```python
from build123d import *

# Parameters (mm, degrees)
SKETCH1_R           = 292.1
BOSS_EXTRUDE1_DEPTH = 127
FILLET1_R           = 38.1
SKETCH2_R           = 15.875
CUT_EXTRUDE1_DEPTH  = 128


with BuildPart() as part:
    # Sketch1 → Boss-Extrude1 (new body)
    with BuildSketch(Plane(origin=(0, 0, 0), x_dir=(1, 0, 0), z_dir=(0, 1, 0))):
        Circle(SKETCH1_R)
    extrude(amount=BOSS_EXTRUDE1_DEPTH)

    # Fillet1
    fillet1_edges = [part.edges().sort_by_distance(p)[0] for p in [
        (-292.1, 0, 0),
        (-292.1, 127, 0),
    ]]
    fillet(fillet1_edges, radius=FILLET1_R)

    # Sketch2 → Cut-Extrude1 (cut, through all)
    with BuildSketch(Plane(origin=(0, 127, 0), x_dir=(1, 0, 0), z_dir=(0, 1, 0))):
        Circle(SKETCH2_R)
    extrude(amount=-CUT_EXTRUDE1_DEPTH, mode=Mode.SUBTRACT)


solid = part.part
```
Geometry: final body of the model. Coordinates: model frame, mm. Coordinates: 2 decimals unless noted, no trailing zeros. Loops run counter-clockwise (first coordinate to the right, second up) from the corner with the lowest first, then second, coordinate; pieces in that order, holes last. Notation, with made-up numbers: M 50,-18 L 64,-18 A11 cw 64,-13 Z; hole C 34.25,6 d3. An arc over 180 degrees is marked long. Put each result on its own line as item: value.
(1) Cut plane A-A on x = 0. Return the cut outline in (y, z) (3 decimals), then the cut area to 3 significant figures.
Answer sheet:
outline: M 0,-254 A38.1 ccw 38.1,-292.1 L 88.9,-292.1 A38.1 ccw 127,-254 L 127,-15.875 L 0,-15.875 Z; M 0,15.875 L 127,15.875 L 127,254 A38.1 ccw 88.9,292.1 L 38.1,292.1 A38.1 ccw 0,254 Z
area: 68,900 mm^2
(2) Cut plane B-B on z = 0. Return the cut outline in (x, y) (3 decimals), then the cut area to 3 significant figures.
Answer sheet:
outline: M -292.1,38.1 A38.1 ccw -254,0 L -15.875,0 L -15.875,127 L -254,127 A38.1 ccw -292.1,88.9 Z; M 15.875,0 L 254,0 A38.1 ccw 292.1,38.1 L 292.1,88.9 A38.1 ccw 254,127 L 15.875,127 Z
area: 68,900 mm^2
(3) First-contact query: pin 1 (10 mm diameter, centred on x = -194, y = 74, fed in from -Z); pin 2 (2 mm diameter, centred on y = 56, z = 137.5, fed in from -X); pin 3 (6 mm diameter, centred on x = -12, z = -71, fed in from -Y); pin 4 (10 mm diameter, centred on y = 60.5, z = -217, fed in from -X). Flat tips, straight axial feed; report the tip coordinate or a pass-through.
Answer sheet:
pin 1: stops at z = -222.71
pin 2: stops at x = -258.24
pin 3: stops at y = 0
pin 4: stops at x = -200.94
(4) Cut plane C-C on y = 61. Return the cut outline in (x, z) (3 decimals), then the cut area to 3 significant figures.
Answer sheet:
outline: C 0,0 d584.2; hole C 0,0 d31.75
area: 267,000 mm^2
(5) Draft query along X for faces 1 (the face through (53, 0, -4)), 2 (the face through (278.61, 63.14, -87.74)), 3 (the face through (-3.441, 64.389, 15.497)). Return one class per face: pulls with the +X half, pulls with the -X half, needs draft (parallel to the pull), parting line crosses it, or undercut.
Answer sheet:
face 1: needs draft
face 2: parting line crosses it
face 3: undercut
(6) Material intervals for probe 1 along Z at (x, y) = (0, 45) (3 decimals); probe 2 along Z at (x, y) = (0, 34) (3 decimals), sorted ascending.
Answer sheet:
probe 1: z = -292.1 to -15.875, 15.875 to 292.1
probe 2: z = -291.879 to -15.875, 15.875 to 291.879
